Answer from the drawing. Dimensions are ordinates in mm from the lowest x, y and z of the part. A direction names the side the tool comes from. Give positions to 0.01 mm unless a question says otherwise; leave off trailing zeros. Write each loop counter-clockwise with the first axis right and the second up, starting at its lowest first coordinate (ties: lowest second). Pieces come first, ordered by that corner, then holes. Notation, with made-up numbers: (-22, 70.25) -> (2, 70.25) arc R20 ccw to (2, 95.25) -> close; hole circle Ø7 at (82, 47). An arc over 180 degrees is marked (long way). Write item = value, one per line.
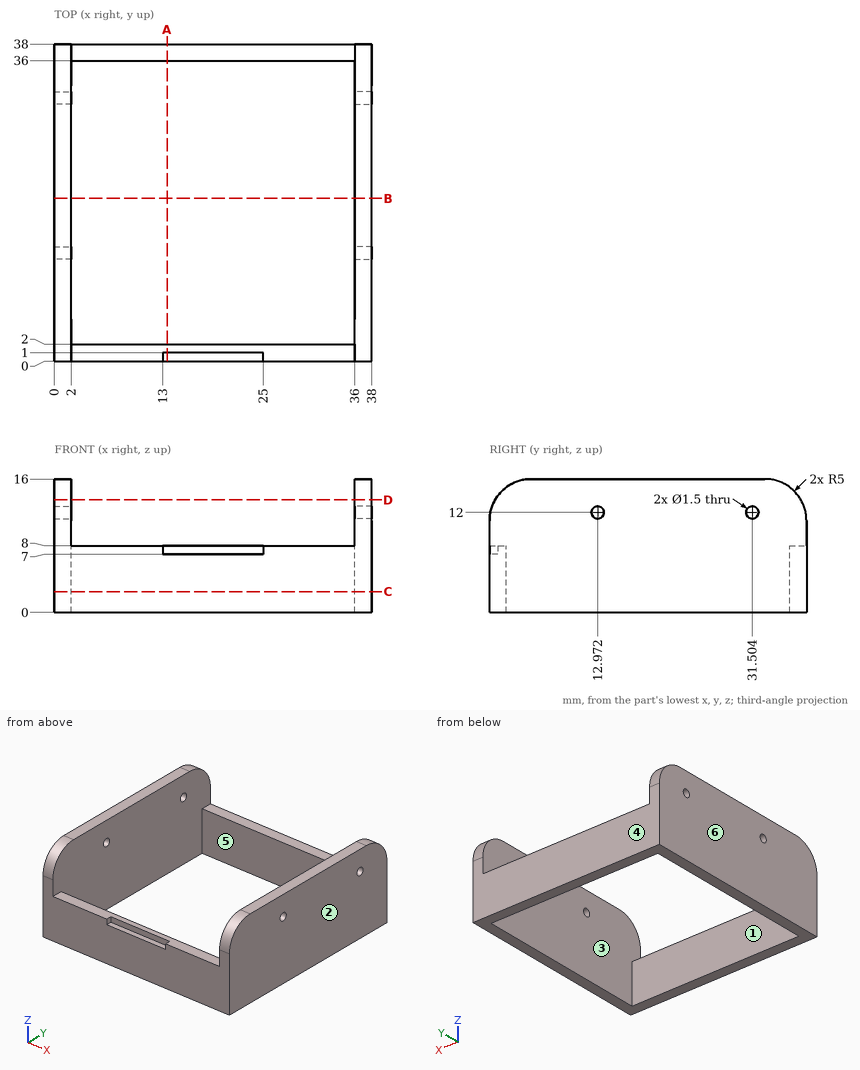
(1) The part is cut by section C-C on z = 2.5. Determine the outline of the cut face in (x, y).
Checks:
outline = (0, 0) -> (38, 0) -> (38, 38) -> (0, 38) -> close; hole (2, 2) -> (36, 2) -> (36, 36) -> (2, 36) -> close
(2) The part is cut by section A-A on x = 13.5. Determine the outline of the cut face in (y, z), plus the area to 3 significant figures.
Checks:
outline = (0, 0) -> (2, 0) -> (2, 8) -> (1, 8) -> (1, 7) -> (0, 7) -> close; (36, 0) -> (38, 0) -> (38, 8) -> (36, 8) -> close
area = 31.0 mm²
(3) The part is cut by section D-D on z = 13.5. Determine the outline of the cut face in (x, y), plus the area to 3 significant figures.
Checks:
outline = (0, 0.67) -> (2, 0.67) -> (2, 37.33) -> (0, 37.33) -> close; (36, 0.67) -> (38, 0.67) -> (38, 37.33) -> (36, 37.33) -> close
area = 147 mm²
(4) The part is cut by section B-B on y = 19.5. Determine the outline of the cut face in (x, z), plus the area to 3 significant figures.
Checks:
outline = (0, 0) -> (2, 0) -> (2, 16) -> (0, 16) -> close; (36, 0) -> (38, 0) -> (38, 16) -> (36, 16) -> close
area = 64.0 mm²
(5) A tool of negligible diameter and unlimited length cuts with its end or side. For the marked faces 1 and 2, from which of +Z, -Z, +X, -X, +Y, -Y can it reach the whole face along a straight path? Write none if from no direction.
Checks:
face_1 = +Z, -Z
face_2 = +Z, -Z, +X, +Y, -Y
(6) Consider L1, parallel to Y at x = 29.5, z = 3.5; L2, parallel to Y at x = 23.5, z = 7.75. Determine where each line is inside the solid, lowest interval first.
Checks:
L1 = 0 to 2, 36 to 38
L2 = 1 to 2, 36 to 38
(7) For a pull along X with two mould halves and no side action, classify the marked faces 3, 4, 5 and 6 as released by +X, released by -X, zero draft, split by the parting line, or undercut.
Checks:
face_3 = undercut
face_4 = zero draft
face_5 = undercut
face_6 = released by -X
(8) Given P1, Ø0.6, axis at x = 18, y = 0.5, coming from the +Z side; P2, Ø1.6, axis at x = 10.5, y = 37, coming from the +Z side, each flat-ended and moving along its own axis, determine where each tip first touches the part or whether it passes through.
Checks:
P1 = 7
P2 = 8
